Geometry: final body of the model. Coordinates: model frame, mm. A direction names the side the tool comes from. Give positions to 0.01 mm unless a question says otherwise; leave off trailing zeros. Write each loop counter-clockwise with the first axis right and the second up, starting at its lowest first coordinate (ties: lowest second). Pieces come first, ordered by that corner, then holes.
from build123d import *

# Parameters (mm, degrees)
ESQUISSE1_W             = 100
ESQUISSE1_H             = 65
BOSS_EXTRU_1_DEPTH      = 5
ESQUISSE2_W             = 15
ESQUISSE2_H             = 5.01
ESQUISSE2_W_2           = 15.01
ESQUISSE2_W_3           = 14.51
ESQUISSE2_H_2           = 5
ESQUISSE2_W_4           = 5
ESQUISSE2_H_3           = 17.5
ENL_V_MAT_EXTRU_1_DEPTH = 5
ESQUISSE7_R             = 9.505
ENL_V_MAT_EXTRU_5_DEPTH = 10
ENL_V_MAT_EXTRU_6_DEPTH = 10


with BuildPart() as part:
    # Esquisse1 → Boss.-Extru.1 (new body)
    with BuildSketch(Plane.XY):
        Rectangle(ESQUISSE1_W, ESQUISSE1_H)
    extrude(amount=BOSS_EXTRU_1_DEPTH)

    # Esquisse2 → Enlèv. mat.-Extru.1 (cut)
    with BuildSketch(Plane.XY.offset(5)):
        with Locations((-42.5, 29.995)):
            Rectangle(ESQUISSE2_W, ESQUISSE2_H)
        with Locations((-14.005, 29.995)):
            Rectangle(ESQUISSE2_W_2, ESQUISSE2_H)
        with Locations((14.495, 29.995)):
            Rectangle(ESQUISSE2_W_2, ESQUISSE2_H)
        with Locations((42.745, 30)):
            Rectangle(ESQUISSE2_W_3, ESQUISSE2_H_2)
        with Locations((-47.5, 0.25)):
            Rectangle(ESQUISSE2_W_4, ESQUISSE2_H_3)
        with Locations((47.5, 0.25)):
            Rectangle(ESQUISSE2_W_4, ESQUISSE2_H_3)
        with Locations((42.745, -30)):
            Rectangle(ESQUISSE2_W_3, ESQUISSE2_H_2)
        with Locations((14.495, -29.995)):
            Rectangle(ESQUISSE2_W_2, ESQUISSE2_H)
        with Locations((-14.005, -29.995)):
            Rectangle(ESQUISSE2_W_2, ESQUISSE2_H)
        with Locations((-42.5, -29.995)):
            Rectangle(ESQUISSE2_W, ESQUISSE2_H)
    extrude(amount=-ENL_V_MAT_EXTRU_1_DEPTH, mode=Mode.SUBTRACT)

    # Esquisse7 → Enlèv. mat.-Extru.5 (cut)
    with BuildSketch(Plane.XY.offset(5)):
        with Locations((-12, -13)):
            Circle(ESQUISSE7_R)
    extrude(amount=-ENL_V_MAT_EXTRU_5_DEPTH, mode=Mode.SUBTRACT)

    # Esquisse8 → Enlèv. mat.-Extru.6 (cut)
    with BuildSketch(Plane.XY.offset(5)):
        with BuildLine():
            Line((24.87958624, -0.692121258), (19.479698297, -3.30769198))
            ThreePointArc((19.479698297, -3.30769198), (12.800149409, -0.98742763), (15.12041376, 5.692121258))
            Line((15.12041376, 5.692121258), (20.520301703, 8.30769198))
            ThreePointArc((20.520301703, 8.30769198), (27.199850591, 5.98742763), (24.87958624, -0.692121258))
        make_face()
        with BuildLine():
            Line((23.353836652, 14.707813375), (17.953948709, 12.092242653))
            ThreePointArc((17.953948709, 12.092242653), (15.950084043, 12.788321958), (16.646163348, 14.792186625))
            Line((16.646163348, 14.792186625), (22.046051291, 17.407757347))
            ThreePointArc((22.046051291, 17.407757347), (24.049915957, 16.711678042), (23.353836652, 14.707813375))
        make_face()
        with BuildLine():
            Line((23.353836652, -9.792186625), (17.953948709, -12.407757347))
            ThreePointArc((17.953948709, -12.407757347), (15.950084043, -11.711678042), (16.646163348, -9.707813375))
            Line((16.646163348, -9.707813375), (22.046051291, -7.092242653))
            ThreePointArc((22.046051291, -7.092242653), (24.049915957, -7.788321958), (23.353836652, -9.792186625))
        make_face()
        with BuildLine():
            Line((11.103836652, 2.457813375), (5.703948709, -0.157757347))
            ThreePointArc((5.703948709, -0.157757347), (3.700084043, 0.538321958), (4.396163348, 2.542186625))
            Line((4.396163348, 2.542186625), (9.796051291, 5.157757347))
            ThreePointArc((9.796051291, 5.157757347), (11.799915957, 4.461678042), (11.103836652, 2.457813375))
        make_face()
        with BuildLine():
            Line((35.603836652, 2.457813375), (30.203948709, -0.157757347))
            ThreePointArc((30.203948709, -0.157757347), (28.200084043, 0.538321958), (28.896163348, 2.542186625))
            Line((28.896163348, 2.542186625), (34.296051291, 5.157757347))
            ThreePointArc((34.296051291, 5.157757347), (36.299915957, 4.461678042), (35.603836652, 2.457813375))
        make_face()
    extrude(amount=-ENL_V_MAT_EXTRU_6_DEPTH, mode=Mode.SUBTRACT)


solid = part.part
Q1. Ray query, line 1 along Y through (x, z) = (-12, 2.6) (3 decimals); line 2 along X through (y, z) = (29.5, 1.2); line 3 along X through (y, z) = (-8, 0.8). Return the intervals inside material, ascending.
Filled sheet:
line 1: y = -27.49 to -22.505, -3.495 to 27.49
line 2: x = -35 to -21.51, -6.5 to 6.99, 22 to 35.49
line 3: x = -45 to -20.08, -3.92 to 20.17, 24.13 to 45
Q2. Section A-A on x = -12. Output: boundary loops of the cut face in (y, z) (3 decimals).
Filled sheet:
outline: (-27.49, 0) - (-22.505, 0) - (-22.505, 5) - (-27.49, 5) - close; (-3.495, 0) - (27.49, 0) - (27.49, 5) - (-3.495, 5) - close
Q3. Pull-direction query (Y, two-part tool) for faces 1 (the cylindrical face through (15.965, 12.759, 2.535)), 2 (the flat face through (-50, 18, 2)), 3 (the flat face through (29, -32.5, 2)); classes: released by +Y, released by -Y, zero draft, split by the parting line, or undercut.
Filled sheet:
face 1: undercut
face 2: zero draft
face 3: released by -Y
Q4. Access query for faces 4 (the flat face through (32.942, 1.168, 2.535)), 5 (the flat face through (22, 30, 3)), 6 (the flat face through (43, 27.5, 3)), 7 (the flat face through (-48, 9, 3)), 8 (the flat face through (-35, -30, 3)). Directions: +Z, -Z, +X, -X, +Y, -Y. A direction counts if a zero-diameter tool reaches every point of the face in a straight line with its end or side. Return the directions, or none.
Filled sheet:
face 4: +Z, -Z
face 5: +Z, -Z, +Y
face 6: +Z, -Z, +X, +Y
face 7: +Z, -Z, -X
face 8: +Z, -Z, -X, -Y
Q5. Pin query (flat end, axial travel): P1, Ø1.5, axis at x = 11, z = 3, coming from the +Y side; P2, Ø2.5, axis at y = -29, z = 1.5, coming from the -X side; P3, Ø1.5, axis at y = -2.5, z = 1.5, coming from the -X side; P4, Ø6, axis at x = -14, y = -17.5, coming from the +Z side. Return the tip coordinate at first contact, or that it passes through.
Filled sheet:
P1: stops at y = 27.49
P2: stops at x = -35
P3: stops at x = -45
P4: passes through
Q6. Section B-B on z = 1.15. Count the separate pieces of the cut face and the enclosed holes in it, plus the area to 3 significant figures.
Filled sheet:
separate pieces: 1
enclosed holes: 6
area: 5,210 mm2
